from build123d import *

# Parameters (mm, degrees)
F0_W     = 96.733004
F0_H     = 52.915374
F1_DEPTH = 28.956
F2_R     = 14.838467
F3_DEPTH = 5.842
F4_R     = 7.671079
F5_DEPTH = 1.524


with BuildPart() as f1:
    # F0 (on Front) → F1 (new body)
    with BuildSketch(Plane.XZ):
        with Locations((-48.366502, 18.087014)):
            Rectangle(F0_W, F0_H)
    extrude(amount=F1_DEPTH)

    # F2 (on face) → F3 (join)
    with BuildSketch(Plane.XZ.offset(28.956)):
        with Locations((-73.99255, 19.509472)):
            Circle(F2_R)
    extrude(amount=F3_DEPTH)

    # F4 (on face) → F5 (join)
    with BuildSketch(Plane.XY.offset(44.544701)):
        with Locations((-80.607049, -16.305355)):
            Circle(F4_R)
    extrude(amount=F5_DEPTH)


solid = f1.part
Work out the finished part from the listing and answer in its coordinate system (mm). A direction names the side the tool comes from. Coordinates: 2 decimals unless noted, no trailing zeros. Write each loop counter-clockwise with the first axis right and the second up, starting at its lowest first coordinate (ties: lowest second). Pieces come first, ordered by that corner, then holes.
1. The part is cut by section A-A, the plane x = -64. Write down the section's boundary in (y, z), and give its area (3 significant figures).
Results list:
outline: (-34.8, 8.54) - (-28.96, 8.54) - (-28.96, -8.37) - (0, -8.37) - (0, 44.54) - (-28.96, 44.54) - (-28.96, 30.48) - (-34.8, 30.48) - close
area: 1,660 mm2
2. The part is cut by section B-B, the plane z = 30.5. Write down the section's boundary in (x, y).
Results list:
outline: (-96.73, -28.96) - (-83.96, -28.96) - (-83.96, -34.8) - (-64.02, -34.8) - (-64.02, -28.96) - (0, -28.96) - (0, 0) - (-96.73, 0) - close
3. The part is cut by section D-D, the plane z = 3.5. Write down the section's boundary in (x, y), and give its area (3 significant figures).
Results list:
outline: (-96.73, -28.96) - (0, -28.96) - (0, 0) - (-96.73, 0) - close
area: 2,800 mm2
4. Flat-ended cylindrical pins translate along their axes: pin 1 (5 mm diameter, centred on x = -69.5, y = -28.5, fed in from +Z); pin 2 (12 mm diameter, centred on x = -25, z = 40.5, fed in from -Y). Find the tip coordinate at first contact, or state that the pin passes through.
Results list:
pin 1: stops at z = 44.54
pin 2: stops at y = -28.96
5. Consider line 1 along Y through (x, z) = (-39.5, 34); line 2 along Z through (x, y) = (-9, -27.5); line 3 along X through (y, z) = (-32, 7.5). Determine where each line is inside the solid, lowest interval first.
Results list:
line 1: y = -28.96 to 0
line 2: z = -8.37 to 44.54
line 3: x = -82.71 to -65.28
6. For faces 1 (the cylindrical face through (-77.067, -23.111, 45.296)), 2 (the flat face through (-49, 0, 18)), 3 (the cylindrical face through (-88.817, -31.836, 20.162)), determine the directions among +Z, -Z, +X, -X, +Y, -Y from which every point of the face is accessible in a straight line to the end or side of a thin tool.
Results list:
face 1: +Z
face 2: +Z, -Z, +X, -X, +Y
face 3: -Y
7. The part is cut by section C-C, the plane y = -7. Write down the section's boundary in (x, z), and give its area (3 significant figures).
Results list:
outline: (-96.73, -8.37) - (0, -8.37) - (0, 44.54) - (-96.73, 44.54) - close
area: 5,120 mm2
